from build123d import *

# Parameters (mm, degrees)
CROQUIS1_W              = 1258.2
CROQUIS1_H              = 1300
SALIENTE_EXTRUIR1_DEPTH = 2.9
CROQUIS2_W              = 800
CROQUIS2_H              = 550
CORTAR_EXTRUIR1_DEPTH   = 2.9
CROQUIS3_W              = 430
CROQUIS3_H              = 135
CORTAR_EXTRUIR2_DEPTH   = 10


with BuildPart() as part:
    # Croquis1 → Saliente-Extruir1 (new body)
    with BuildSketch(Plane.XY):
        with Locations((629.1, -650)):
            Rectangle(CROQUIS1_W, CROQUIS1_H)
    extrude(amount=SALIENTE_EXTRUIR1_DEPTH)

    # Croquis2 → Cortar-Extruir1 (cut)
    with BuildSketch(Plane.XY.offset(2.9)):
        with Locations((629.1, -1025)):
            Rectangle(CROQUIS2_W, CROQUIS2_H)
    extrude(amount=-CORTAR_EXTRUIR1_DEPTH, mode=Mode.SUBTRACT)

    # Croquis3 → Cortar-Extruir2 (cut)
    with BuildSketch(Plane.XY.offset(2.9)):
        with Locations((473, -67.5)):
            Rectangle(CROQUIS3_W, CROQUIS3_H)
    extrude(amount=-CORTAR_EXTRUIR2_DEPTH, mode=Mode.SUBTRACT)


solid = part.part
Geometry check sheet. Reference: the model listing, model coordinates, mm. Give positions to 0.01 mm unless a question says otherwise; leave off trailing zeros. Order: outer loops, then holes, each group sorted by start corner. A loop starts at its lowest first (then second) coordinate and runs counter-clockwise, first axis right, second up.
1) Cross-section at D-D (x = 492.5). Record the boundary of the cut face in (y, z).
Results are:
outline: (-750, 0) - (-135, 0) - (-135, 2.9) - (-750, 2.9) - close
2) Cross-section at C-C (x = 1003). Record the boundary of the cut face in (y, z), then the cut area to 4 significant figures.
Results are:
outline: (-750, 0) - (0, 0) - (0, 2.9) - (-750, 2.9) - close
area: 2,175 mm2
3) Cross-section at B-B (z = 0.7). Record the boundary of the cut face in (x, y).
Results are:
outline: (0, -1300) - (229.1, -1300) - (229.1, -750) - (1029.1, -750) - (1029.1, -1300) - (1258.2, -1300) - (1258.2, 0) - (688, 0) - (688, -135) - (258, -135) - (258, 0) - (0, 0) - close
4) Material ranges on probe 1 along X at (y, z) = (-914, 2.1); probe 2 along Y at (x, z) = (700.5, 1.4); probe 3 along Y at (x, z) = (640.5, 1.75), recorded low to high.
Results are:
probe 1: x = 0 to 229.1, 1029.1 to 1258.2
probe 2: y = -750 to 0
probe 3: y = -750 to -135
5) Cross-section at A-A (y = -954). Record the boundary of the cut face in (x, z), then the cut area to 3 significant figures.
Results are:
outline: (0, 0) - (229.1, 0) - (229.1, 2.9) - (0, 2.9) - close; (1029.1, 0) - (1258.2, 0) - (1258.2, 2.9) - (1029.1, 2.9) - close
area: 1,330 mm2
